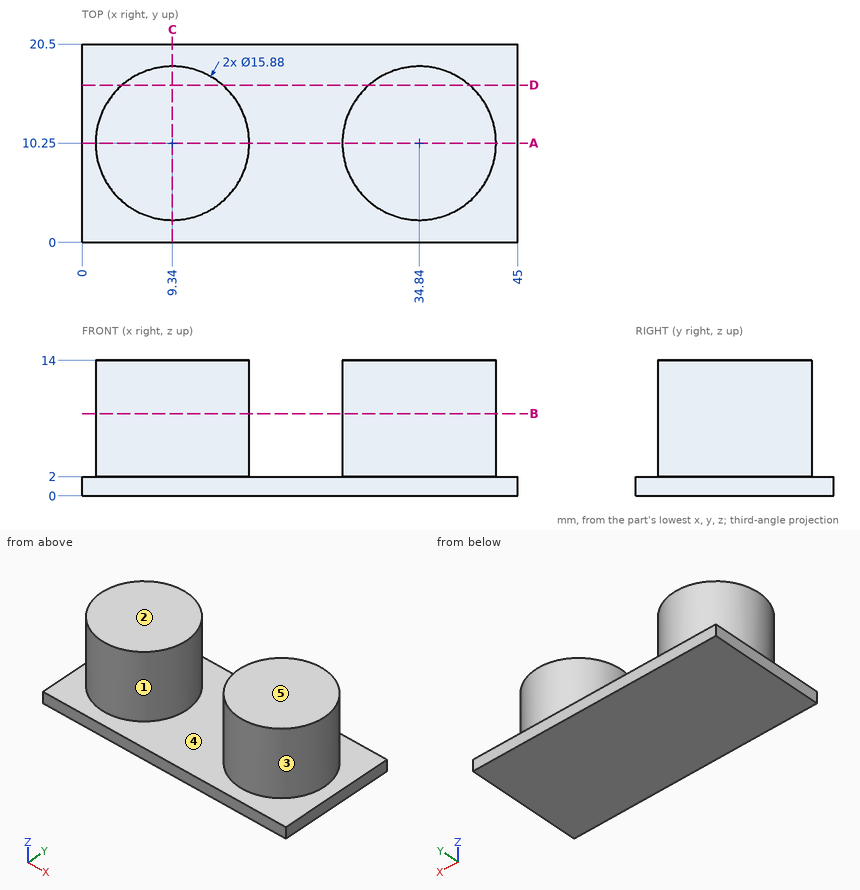
Could you check a few things on this drawing? It's one solid part, dimensions in mm from its lowest x, y, z. A direction names the side the tool comes from. Give positions to 0.01 mm unless a question says otherwise; leave off trailing zeros. Loops run counter-clockwise (first coordinate to the right, second up) from the corner with the lowest first, then second, coordinate; pieces in that order, holes last. Notation, with made-up numbers: M -23,57 L 14,57 A26 ccw 14,94 Z; hole C 28.5,48.25 d5. An arc over 180 degrees is marked long. Answer as a JSON object with one key per item and string values.
Q1. For P1, Ø10, axis at x = 17, y = 14, coming from the +Z side; P2, Ø8, axis at x = 20.5, z = 11, coming from the +Y side; P3, Ø2, axis at y = 9.5, z = 8.5, coming from the +X side; P4, Ø6, axis at x = 36, z = 12.5, coming from the +Y side, each with a flat end and sliding along its axis, tell me the tip position at first contact or that it passes through.
Values found:
{"P1": "stops at z = 14", "P2": "stops at y = 13.68", "P3": "stops at x = 42.78", "P4": "stops at y = 18.19"}
Q2. If I drill on probe 1 along Y at (x, z) = (35, 6.25); probe 2 along X at (y, z) = (4, 6.25); probe 3 along X at (y, z) = (15.5, 10.25), over which ranges is the centre line in solid material (lowest first)? Write a range as [from, to].
Values found:
{"probe 1": "y = [2.31, 18.19]", "probe 2": "x = [4.44, 14.24], [29.94, 39.74]", "probe 3": "x = [3.38, 15.3], [28.88, 40.8]"}
Q3. Suppose I cut it at A-A, the plane y = 10.25. List the corners of the cut face in (x, z) for me.
Values found:
{"outline": "M 0,0 L 45,0 L 45,2 L 42.78,2 L 42.78,14 L 26.9,14 L 26.9,2 L 17.28,2 L 17.28,14 L 1.4,14 L 1.4,2 L 0,2 Z"}
Q4. For the marked faces 4 and 5, which set-ups out of +Z, -Z, +X, -X, +Y, -Y let a thin tool reach every point of the face, with its end or its side?
Values found:
{"face 4": "+Z", "face 5": "+Z, +X, -X, +Y, -Y"}
Q5. Suppose I cut it at B-B, the plane z = 8.5. List the corners of the cut face in (x, y) for me.
Values found:
{"outline": "C 9.34,10.25 d15.88; C 34.84,10.25 d15.88"}
Q6. Suppose I cut it at D-D, the plane y = 16.25. List the corners of the cut face in (x, z) for me, plus the area to 3 significant figures.
Values found:
{"outline": "M 0,0 L 45,0 L 45,2 L 40.04,2 L 40.04,14 L 29.64,14 L 29.64,2 L 14.54,2 L 14.54,14 L 4.14,14 L 4.14,2 L 0,2 Z", "area": "340 mm²"}
Q7. Suppose I cut it at C-C, the plane x = 9.34. List the corners of the cut face in (y, z) for me.
Values found:
{"outline": "M 0,0 L 20.5,0 L 20.5,2 L 18.19,2 L 18.19,14 L 2.31,14 L 2.31,2 L 0,2 Z"}
Q8. If we mould it in two halves opening along X, with no side actions, what happens to the marked faces 1, 2 and 3? For each: pulls with the +X half, pulls with the -X half, needs draft (parallel to the pull), parting line crosses it, or undercut.
Values found:
{"face 1": "undercut", "face 2": "needs draft", "face 3": "undercut"}
